from build123d import *

# Parameters (mm, degrees)
SKETCH3_W           = 20
SKETCH3_H           = 20
BOSS_EXTRUDE2_DEPTH = 20
SKETCH1_W           = 80
SKETCH1_H           = 10
BOSS_EXTRUDE3_DEPTH = 10
SKETCH6_W           = 5
SKETCH6_H           = 30
BOSS_EXTRUDE4_DEPTH = 10


with BuildPart() as part:
    # Sketch3 → Boss-Extrude2 (new body)
    with BuildSketch(Plane(origin=(0, 0, 0), x_dir=(1, 0, 0), z_dir=(0, 1, 0))):
        with Locations((48.654441815, 0)):
            Rectangle(SKETCH3_W, SKETCH3_H)
    extrude(amount=BOSS_EXTRUDE2_DEPTH)

    # Sketch1 → Boss-Extrude3 (add)
    with BuildSketch(Plane(origin=(0, 0, 0), x_dir=(1, 0, 0), z_dir=(0, 1, 0))):
        Rectangle(SKETCH1_W, SKETCH1_H)
    extrude(amount=BOSS_EXTRUDE3_DEPTH)

    # Sketch6 → Boss-Extrude4 (add)
    with BuildSketch(Plane(origin=(0, 0, 0), x_dir=(1, 0, 0), z_dir=(0, 1, 0))):
        with Locations((-37.345197049, -20)):
            Rectangle(SKETCH6_W, SKETCH6_H)
    extrude(amount=BOSS_EXTRUDE4_DEPTH)


solid = part.part
Verification items for the finished model (mm, model axes). A direction names the side the tool comes from. Coordinates: 2 decimals unless noted, no trailing zeros. Write each loop counter-clockwise with the first axis right and the second up, starting at its lowest first coordinate (ties: lowest second). Pieces come first, ordered by that corner, then holes. Notation, with made-up numbers: (-15, 11) -> (33, 11) arc R25 cw to (33, 48) -> close; hole circle Ø1 at (-6, -22). An arc over 180 degrees is marked (long way). One line per item, written item: value. Start each with the question number.
Q1. Mould release check, pull along X, two halves, no side actions. Record for faces 4 (the flat face through (38.654, 12, 0)), 5 (the flat face through (1, 5, 5)), 6 (the flat face through (49, 10, 10)), 7 (the flat face through (-39.845, 5, 20)): pulls with the +X half, pulls with the -X half, needs draft (parallel to the pull), parting line crosses it, or undercut.
Q2. Cross-section at B-B on z = 0. Enter the section's corners in (x, y), and give its area (3 significant figures).
Q3. Access from +Z, -Z, +X, -X, +Y, -Y to the whole of each face (thin tool, end or side, straight path). Record for faces 1 (the flat face through (-1, 5, -5)), 2 (the flat face through (49, 20, 0)), 3 (the flat face through (-6.7, 10, 4.5)).
Q4. Cross-section at A-A on y = 5.5. Enter the section's corners in (x, z), and give its area (3 significant figures).
Q5. Go/stop test with flat-tipped pins: P1, Ø11, axis at y = 4, z = 27, coming from the -X side; P2, Ø6, axis at x = -1, z = -2.5, coming from the -Y side; P3, Ø10, axis at x = -16.5, y = 4, coming from the -Z side; P4, Ø6, axis at x = 44, y = 14, coming from the +Z side. Record where each tip stops, or that it passes through.
Q6. Thickness scan on L1, parallel to Z at x = -1, y = 7.5; L2, parallel to Z at x = 46, y = 5.75; L3, parallel to X at y = 1.25, z = 10.5. Record the ranges inside material, lowest first. Write a range as from..to.
Q7. Cross-section at C-C on x = 48. Enter the section's corners in (y, z), and give its area (3 significant figures).
Q8. Cross-section at D-D on z = 23. Enter the section's corners in (x, y), and give its area (3 significant figures).
Checked values:
1. face 4: undercut
1. face 5: undercut
1. face 6: needs draft
1. face 7: pulls with the -X half
2. outline: (-40, 0) -> (58.65, 0) -> (58.65, 20) -> (38.65, 20) -> (38.65, 10) -> (-40, 10) -> close
2. area: 1,190 mm²
3. face 1: -Z, -X, +Y, -Y
3. face 2: +Z, -Z, +X, -X, +Y
3. face 3: +Z, -Z, -X, +Y
4. outline: (-40, -5) -> (38.65, -5) -> (38.65, -10) -> (58.65, -10) -> (58.65, 10) -> (38.65, 10) -> (38.65, 5) -> (-34.85, 5) -> (-34.85, 35) -> (-39.85, 35) -> (-39.85, 5) -> (-40, 5) -> close
4. area: 1,340 mm²
5. P1: stops at x = -39.85
5. P2: stops at y = 0
5. P3: stops at z = -5
5. P4: stops at z = 10
6. L1: z = -5..5
6. L2: z = -10..10
6. L3: x = -39.85..-34.85
7. outline: (0, -10) -> (20, -10) -> (20, 10) -> (0, 10) -> close
7. area: 400 mm²
8. outline: (-39.85, 0) -> (-34.85, 0) -> (-34.85, 10) -> (-39.85, 10) -> close
8. area: 50.0 mm²
